Here's how the part is built. I have some questions about the finished solid (model axes, mm). Face numbers are marked on the shaded views. Give positions to 0.01 mm unless a question says otherwise; leave off trailing zeros. Write each loop counter-clockwise with the first axis right and the second up, starting at its lowest first coordinate (ties: lowest second). Pieces come first, ordered by that corner, then holes. Notation, with made-up numbers: (44, 64) -> (58, 64) arc R25 cw to (58, 91) -> close; hole circle Ø8 at (45, -7). An arc over 180 degrees is marked (long way). Use CSV: the item, a comma, the result in double quotes. Start each with the question number.
(1) Suppose I cut it at A-A on z = 5. List the corners of the cut face in (x, y) for me, plus the area to 3 significant figures.
(2) I need wall thicknesses on L1, parallel to X at y = 2.65, z = 5; L2, parallel to Y at x = 5.5, z = 0.75; L3, parallel to X at y = 6.25, z = 1. Which ranges of each line are inside material? Lowest first, please. Write a range as [from, to].
(3) For pin 1 Ø5.5 at (x, z) = (5, 5) entering from -Y, with a flat end and sliding along its axis, tell me the tip position at first contact or that it passes through.
(4) Suppose I cut it at C-C on y = 2.25. List the corners of the cut face in (x, z) for me.
(5) Suppose I cut it at D-D on y = 13. List the corners of the cut face in (x, z) for me, plus the area to 3 significant figures.
(6) Suppose I cut it at B-B on x = 5. List the corners of the cut face in (y, z) for me.
(7) If we mould it in two halves opening along X, with no side actions, what happens to the marked faces 1, 2, 3 and 4? For each: pulls with the +X half, pulls with the -X half, needs draft (parallel to the pull), parting line crosses it, or undercut.
from build123d import *

# Parameters (mm, degrees)
SKETCH1_W           = 10
SKETCH1_H           = 10
SKETCH1_R           = 4.5
BOSS_EXTRUDE1_DEPTH = 14.7
SKETCH2_W           = 10
SKETCH2_H           = 10
SKETCH2_R           = 3.5
BOSS_EXTRUDE2_DEPTH = 3
SKETCH3_R           = 4.5
CUT_EXTRUDE1_DEPTH  = 2


with BuildPart() as part:
    # Sketch1 → Boss-Extrude1 (new body)
    with BuildSketch(Plane(origin=(0, 0, 0), x_dir=(1, 0, 0), z_dir=(0, 1, 0))):
        with Locations((5, -5)):
            Rectangle(SKETCH1_W, SKETCH1_H)
        with Locations((5, -5)):
            Circle(SKETCH1_R, mode=Mode.SUBTRACT)
    extrude(amount=BOSS_EXTRUDE1_DEPTH)

    # Sketch2 → Boss-Extrude2 (add)
    with BuildSketch(Plane(origin=(0, 0, 0), x_dir=(-1, 0, 0), z_dir=(0, -1, 0))):
        with Locations((-5, -5)):
            Rectangle(SKETCH2_W, SKETCH2_H)
        with Locations((-5, -5)):
            Circle(SKETCH2_R, mode=Mode.SUBTRACT)
    extrude(amount=-BOSS_EXTRUDE2_DEPTH)

    # Sketch3 → Cut-Extrude1 (cut)
    with BuildSketch(Plane(origin=(0, 0, 0), x_dir=(-1, 0, 0), z_dir=(0, -1, 0))):
        with Locations((-5, -5)):
            Circle(SKETCH3_R)
    extrude(amount=-CUT_EXTRUDE1_DEPTH, mode=Mode.SUBTRACT)


solid = part.part
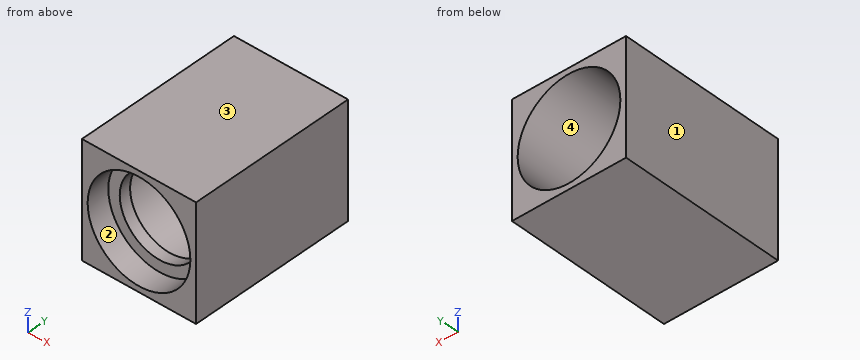
Geometry says:
1,outline,"(0, 0) -> (0.5, 0) -> (0.5, 2) -> (1.5, 2) -> (1.5, 3) -> (0.5, 3) -> (0.5, 14.7) -> (0, 14.7) -> close; (8.5, 2) -> (9.5, 2) -> (9.5, 0) -> (10, 0) -> (10, 14.7) -> (9.5, 14.7) -> (9.5, 3) -> (8.5, 3) -> close"
1,area,"16.7 mm²"
2,L1,"[0, 1.5], [8.5, 10]"
2,L2,"[2, 3]"
2,L3,"[0, 2.94], [7.06, 10]"
3,pin 1,"through"
4,outline,"(0, 0) -> (10, 0) -> (10, 10) -> (0, 10) -> close; hole circle Ø7 at (5, 5)"
5,outline,"(0, 0) -> (10, 0) -> (10, 10) -> (0, 10) -> close; hole circle Ø9 at (5, 5)"
5,area,"36.4 mm²"
6,outline,"(0, 0) -> (14.7, 0) -> (14.7, 0.5) -> (3, 0.5) -> (3, 1.5) -> (2, 1.5) -> (2, 0.5) -> (0, 0.5) -> close; (0, 9.5) -> (2, 9.5) -> (2, 8.5) -> (3, 8.5) -> (3, 9.5) -> (14.7, 9.5) -> (14.7, 10) -> (0, 10) -> close"
7,face 1,"pulls with the -X half"
7,face 2,"undercut"
7,face 3,"needs draft"
7,face 4,"undercut"
